```python
from build123d import *


with BuildPart() as part:
    # Sketch1 → Revolve1 (revolve)
    with BuildSketch(Plane.XY, mode=Mode.PRIVATE) as revolve1_sk:
        Polygon((18.7325, 22.5298), (6.0325, 22.5298), (6.0325, 0), (32.1945, 0), (32.1945, 7.62), (18.7325, 7.62), align=None)
        with BuildLine():
            Line((32.1945, 0), (6.0325, 0))
            Line((6.0325, 0), (6.0325, -23.9268))
            Line((6.0325, -23.9268), (34.1376, -23.9268))
            ThreePointArc((34.1376, -23.9268), (35.933651224, -23.182851224), (36.6776, -21.3868))
            Line((36.6776, -21.3868), (36.6776, -2.54))
            ThreePointArc((36.6776, -2.54), (35.933651224, -0.743948776), (34.1376, 0))
            Line((34.1376, 0), (32.1945, 0))
        make_face()
    revolve(revolve1_sk.sketch.rotate(Axis((0, 0, 0), (0, 1, 0)), 90), axis=Axis((0, 0, 0), (0, 1, 0)))


solid = part.part
```
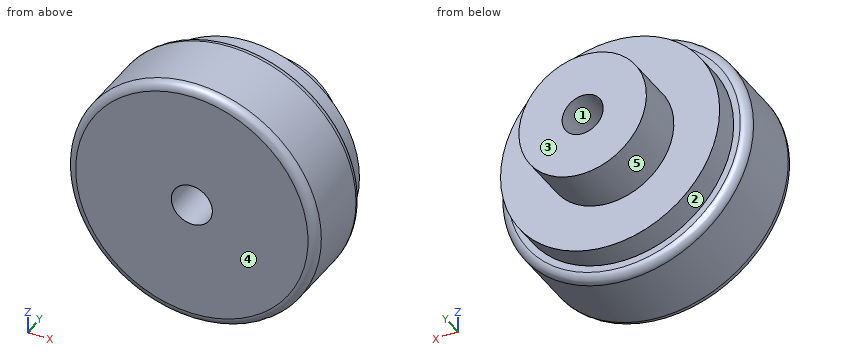
Geometry check sheet. Reference: the model listing, model coordinates, mm. Face numbers are marked on the shaded views. A direction names the side the tool comes from. Round coordinates to 2 decimals unless told otherwise and drop trailing zeros. Write each loop counter-clockwise with the first axis right and the second up, starting at its lowest first coordinate (ties: lowest second). Pieces come first, ordered by that corner, then holes. Notation, with made-up numbers: (22, 67) -> (60, 67) arc R18 cw to (60, 77) -> close; hole circle Ø10 at (-37.75, 2). An arc over 180 degrees is marked (long way). Put each result on its own line as item: value.
1) Release check for a two-part mould opening along X. For the marked faces 1, 2 and 3 record: pulls with the +X half, pulls with the -X half, needs draft (parallel to the pull), parting line crosses it, or undercut.
Recorded:
face 1: undercut
face 2: parting line crosses it
face 3: needs draft
2) Access from +Z, -Z, +X, -X, +Y, -Y to the whole of each face (thin tool, end or side, straight path). Record for the marked faces 4 and 5.
Recorded:
face 4: +Z, -Z, +X, -X, -Y
face 5: +Y
3) Cross-section at B-B, the plane x = 0. Enter the section's corners in (y, z).
Recorded:
outline: (-23.93, -34.14) arc R2.54 ccw to (-21.39, -36.68) -> (-2.54, -36.68) arc R2.54 ccw to (0, -34.14) -> (0, -32.19) -> (7.62, -32.19) -> (7.62, -18.73) -> (22.53, -18.73) -> (22.53, -6.03) -> (-23.93, -6.03) -> close; (-23.93, 6.03) -> (22.53, 6.03) -> (22.53, 18.73) -> (7.62, 18.73) -> (7.62, 32.19) -> (0, 32.19) -> (0, 34.14) arc R2.54 ccw to (-2.54, 36.68) -> (-21.39, 36.68) arc R2.54 ccw to (-23.93, 34.14) -> close
4) Thickness scan on probe 1 along X at (y, z) = (5, 0); probe 2 along X at (y, z) = (-3.5, 0); probe 3 along Y at (x, z) = (-5, -21.5). Record the ranges inside material, lowest first. Write a range as from..to.
Recorded:
probe 1: x = -32.19..-6.03, 6.03..32.19
probe 2: x = -36.68..-6.03, 6.03..36.68
probe 3: y = -23.93..7.62
5) Cross-section at A-A, the plane z = 0. Enter the section's corners in (x, y), plus the area to 3 significant figures.
Recorded:
outline: (-36.68, -21.39) arc R2.54 ccw to (-34.14, -23.93) -> (-6.03, -23.93) -> (-6.03, 22.53) -> (-18.73, 22.53) -> (-18.73, 7.62) -> (-32.19, 7.62) -> (-32.19, 0) -> (-34.14, 0) arc R2.54 ccw to (-36.68, -2.54) -> close; (6.03, -23.93) -> (34.14, -23.93) arc R2.54 ccw to (36.68, -21.39) -> (36.68, -2.54) arc R2.54 ccw to (34.14, 0) -> (32.19, 0) -> (32.19, 7.62) -> (18.73, 7.62) -> (18.73, 22.53) -> (6.03, 22.53) -> close
area: 2,240 mm2
6) Depth check by flat-ended pin: P1, Ø3, axis at x = 25.5, y = 2, coming from the +Z side; P2, Ø1, axis at x = 29, z = 23.5, coming from the -Y side; P3, Ø3, axis at x = 1.5, y = -1.5, coming from the -Z side; P4, Ø1, axis at y = 4, z = -23, coming from the +X side. Enter the tip coordinate at first touch or a pass-through.
Recorded:
P1: stops at z = 21.46
P2: passes through
P3: stops at z = -36.68
P4: stops at x = 23.03
7) Cross-section at C-C, the plane y = -9. Enter the section's corners in (x, z) (1 decimal), plus the area to 3 significant figures.
Recorded:
outline: circle Ø73.4 at (0, 0); hole circle Ø12.1 at (0, 0)
area: 4,110 mm2
